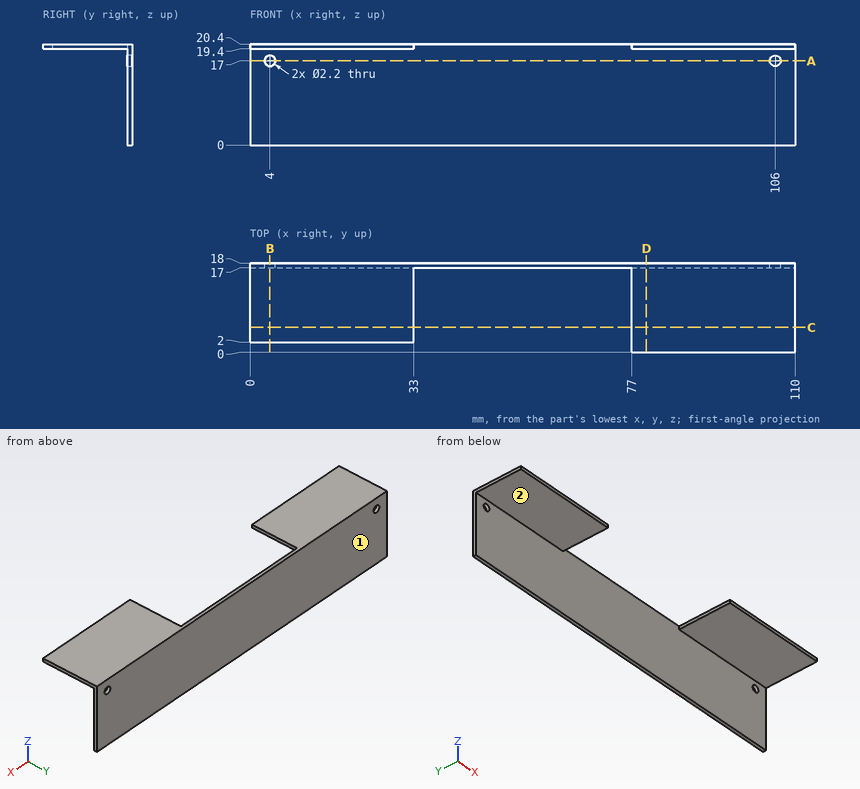
Input: dimensioned drawing with shaded views. Units: mm. Origin: part minimum x, y, z. A direction names the side the tool comes from. Give positions to 0.01 mm unless a question says otherwise; leave off trailing zeros. Order: outer loops, then holes, each group sorted by start corner. A loop starts at its lowest first (then second) coordinate and runs counter-clockwise, first axis right, second up.
(1) Section query C-C (y = 5). Return the cut outline in (x, z).
(2) Section query A-A (z = 17). Return the cut outline in (x, y).
(3) Access query for the marked faces 1 and 2. Directions: +Z, -Z, +X, -X, +Y, -Y. A direction counts if a zero-diameter tool reaches every point of the face in a straight line with its end or side. Return the directions, or none.
(4) Section query D-D (x = 80). Return the cut outline in (y, z), plus the area to 3 significant figures.
(5) Section query B-B (x = 4). Return the cut outline in (y, z), plus the area to 3 significant figures.
(6) Material intervals for line 1 along X through (y, z) = (17.5, 17); line 2 along Z through (x, y) = (4, 17.5); line 3 along Y through (x, z) = (27, 1), sorted ascending.
(7) Contact query for flat-ended pins moving along their axis: P1, Ø1.8, axis at x = 4, z = 17, coming from the +Y side; P2, Ø0.5, axis at x = 12, z = 20, coming from the -Y side; P3, Ø10, axis at x = 87.5, y = 5, coming from the -Z side; P4, Ø6, axis at x = 66, z = 13, coming from the -Y side. Output: stop coordinate, or through.
Outcome:
1. outline: (0, 19.4) - (33, 19.4) - (33, 20.4) - (0, 20.4) - close; (77, 19.4) - (110, 19.4) - (110, 20.4) - (77, 20.4) - close
2. outline: (0, 17) - (2.9, 17) - (2.9, 18) - (0, 18) - close; (5.1, 17) - (104.9, 17) - (104.9, 18) - (5.1, 18) - close; (107.1, 17) - (110, 17) - (110, 18) - (107.1, 18) - close
3. face 1: +Z, -Z, +X, -X, +Y
3. face 2: -Z, +X, -X, -Y
4. outline: (0, 19.4) - (17, 19.4) - (17, 0) - (18, 0) - (18, 20.4) - (0, 20.4) - close
4. area: 37.4 mm2
5. outline: (2, 19.4) - (17, 19.4) - (17, 18.1) - (18, 18.1) - (18, 20.4) - (2, 20.4) - close; (17, 0) - (18, 0) - (18, 15.9) - (17, 15.9) - close
5. area: 33.2 mm2
6. line 1: x = 0 to 2.9, 5.1 to 104.9, 107.1 to 110
6. line 2: z = 0 to 15.9, 18.1 to 20.4
6. line 3: y = 17 to 18
7. P1: passes through
7. P2: stops at y = 2
7. P3: stops at z = 19.4
7. P4: stops at y = 17
